Print and shaded views of the part. All mm, measured from the part's lowest x, y and z. Round coordinates to 2 decimals unless told otherwise and drop trailing zeros. Write each loop counter-clockwise with the first axis right and the second up, starting at its lowest first coordinate (ties: lowest second). Pieces come first, ordered by that corner, then holes.
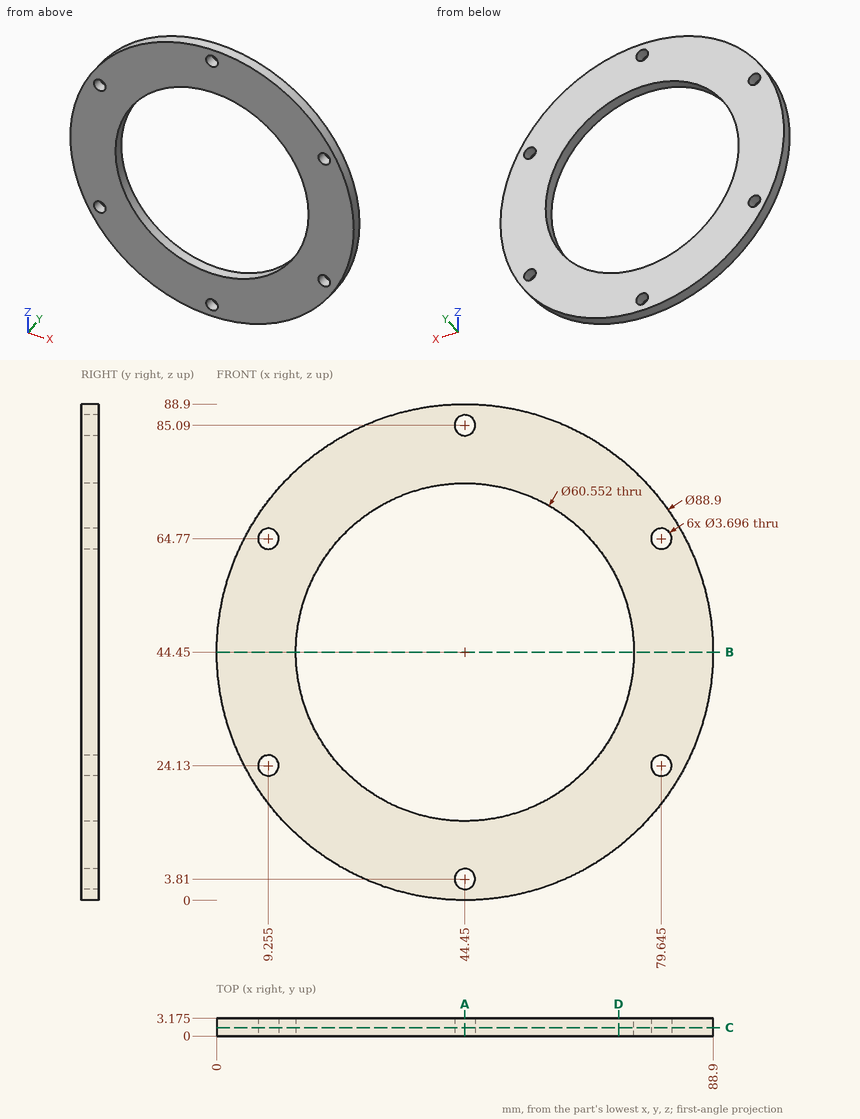
1) Pin check, flat tips, straight feed: pin 1 Ø3.5 at (x, z) = (79.65, 64.77) entering from -Y; pin 2 Ø1 at (y, z) = (1.5, 19) entering from +X. Stop position of each tip, or through.
Results:
pin 1: passes through
pin 2: stops at x = 81.24
2) Slice it at D-D (x = 72). Write the cut outline in (y, z) (1 decimal).
Results:
outline: (0, 9.6) - (3.2, 9.6) - (3.2, 31.9) - (0, 31.9) - close; (0, 57) - (3.2, 57) - (3.2, 79.3) - (0, 79.3) - close
3) Slice it at A-A (x = 44.45). Write the cut outline in (y, z) (1 decimal).
Results:
outline: (0, 0) - (3.2, 0) - (3.2, 2) - (0, 2) - close; (0, 5.7) - (3.2, 5.7) - (3.2, 14.2) - (0, 14.2) - close; (0, 74.7) - (3.2, 74.7) - (3.2, 83.2) - (0, 83.2) - close; (0, 86.9) - (3.2, 86.9) - (3.2, 88.9) - (0, 88.9) - close
4) Wall check: L1, parallel to X at y = 0.6, z = 63.5; L2, parallel to Z at x = 43.5, y = 0.4 (1 decimal); L3, parallel to X at y = 1.8, z = 44.45. Give the ranges that are in metal, low to high.
Results:
L1: x = 4.29 to 7.91, 10.6 to 20.92, 67.98 to 78.3, 80.99 to 84.61
L2: z = 0 to 2.2, 5.4 to 14.2, 74.7 to 83.5, 86.7 to 88.9
L3: x = 0 to 14.17, 74.73 to 88.9
5) Slice it at B-B (z = 44.45). Write the cut outline in (x, y) (1 decimal).
Results:
outline: (0, 0) - (14.2, 0) - (14.2, 3.2) - (0, 3.2) - close; (74.7, 0) - (88.9, 0) - (88.9, 3.2) - (74.7, 3.2) - close
6) Slice it at C-C (y = 1.5). Count the separate pieces of the cut face and the enclosed holes in it, plus the area to 3 significant figures.
Results:
separate pieces: 1
enclosed holes: 7
area: 3,260 mm2
